Could you check a few things on this model? Use its own coordinates, in mm. A direction names the side the tool comes from. Give positions to 0.01 mm unless a question says otherwise; leave off trailing zeros. Loops run counter-clockwise (first coordinate to the right, second up) from the corner with the lowest first, then second, coordinate; pieces in that order, holes last. Notation, with made-up numbers: M 11,-9.5 L 70,-9.5 A8 cw 70,-2.5 Z; hole C 15.5,26.25 d2. An arc over 180 degrees is marked long. Answer in a Markdown table with one row per item. Add a question column.
```python
from build123d import *

# Parameters (mm, degrees)
BOSS_EXTRUDE5_DEPTH      = 6.35
FILLET1_R                = 25.4
CIRPATTERN7_COUNT        = 4
FILLET1_OF_CIRPATTERN7_R = 25.4
SKETCH13_R               = 15.556349186
BOSS_EXTRUDE8_DEPTH      = 6.35
SKETCH1_R                = 5.22699996
SKETCH1_R_2              = 1.686500056
CUT_EXTRUDE1_DEPTH       = 13.7


with BuildPart() as part:
    # Sketch4 → Boss-Extrude5 (new body)
    with BuildSketch(Plane(origin=(0, 0, 0), x_dir=(1, 0, 0), z_dir=(0, 1, 0))):
        Polygon((25.7955, 11), (25.7955, -11), (72.807954542, -58.012454542), (130.820409084, 0), (72.807954542, 58.012454542), align=None)
        Polygon((25.7955, 11), (14.7955, 0), (25.7955, -11), align=None)
        Polygon((25.7955, -11), (14.7955, 0), (25.7955, 11), (0, 11), (0, -11), align=None)
    boss_extrude5 = extrude(amount=BOSS_EXTRUDE5_DEPTH)

    # Fillet1
    fillet1_edges = [part.edges().sort_by_distance(p)[0] for p in [
        (130.820409084, 3.175, 0),
    ]]
    fillet(fillet1_edges, radius=FILLET1_R)

    # CirPattern7: Boss-Extrude5 ×4 about axis
    cirpattern7_axis = Axis((0, 0, 0), (0, 1, 0))
    for i in range(1, CIRPATTERN7_COUNT):
        add(boss_extrude5.rotate(cirpattern7_axis, i * 360 / CIRPATTERN7_COUNT))

    # Fillet1 of CirPattern7
    fillet1_of_cirpattern7_edges = [part.edges().sort_by_distance(p)[0] for p in [
        (0, 3.175, -130.820409084),
        (-130.820409084, 3.175, 0),
        (0, 3.175, 130.820409084),
    ]]
    fillet(fillet1_of_cirpattern7_edges, radius=FILLET1_OF_CIRPATTERN7_R)

    # Sketch13 → Boss-Extrude8 (add)
    with BuildSketch(Plane(origin=(0, 6.35, 0), x_dir=(1, 0, 0), z_dir=(0, 1, 0))):
        Circle(SKETCH13_R)
    extrude(amount=BOSS_EXTRUDE8_DEPTH)

    # Sketch1 → Cut-Extrude1 (cut, through all)
    with BuildSketch(Plane(origin=(0, 0, 0), x_dir=(1, 0, 0), z_dir=(0, 1, 0))):
        Circle(SKETCH1_R)
        with Locations((8.000000002, 0)):
            Circle(SKETCH1_R_2)
        with Locations((0, -8.000000002)):
            Circle(SKETCH1_R_2)
        with Locations((-8.000000002, 0)):
            Circle(SKETCH1_R_2)
        with Locations((0, 8.000000002)):
            Circle(SKETCH1_R_2)
    extrude(amount=CUT_EXTRUDE1_DEPTH, mode=Mode.SUBTRACT)


solid = part.part
```
Item 1: Suppose I cut it at D-D (x = 92.5). List the corners of the cut face in (y, z) for me, then the cut area to 3 significant figures.
Item 2: If we mould it in two halves opening along Z, with no side actions, what happens to faces 3 (the face through (38.27, 3.13, -92.55)), 4 (the face through (-11, 3, 18)), 5 (the face through (7, 12.7, 3))? For each: +Z half, -Z half, draft (parallel to the pull), parting line (faces both ways), or undercut.
Item 3: I need wall thicknesses on L1, parallel to Z at x = 0, y = 6.75; L2, parallel to X at y = 3.75, z = 0. Which ranges of each line are inside material? Lowest first, please.
Item 4: For P1, Ø3, axis at x = -19.5, y = 3.5, coming from the -Z side; P2, Ø5, axis at x = 18.5, y = 4, coming from the +Z side; P3, Ø1.9, axis at y = 3.5, z = 18.5, coming from the +X side; P4, Ø6, axis at x = -36, y = 10.5, coming from the -Z side, each with a flat end and sliding along its axis, tell me the tip position at first contact or that it passes through.
Item 5: Suppose I cut it at B-B (z = -52.5). List the corners of the cut face in (x, y) for me, then the cut area to 3 significant figures.
Item 6: Suppose I cut it at A-A (y = 3.5). Give the number of separate pieces and of enclosed holes in the cut face, then the cut area to 3 significant figures.
Item 7: Suppose I cut it at C-C (x = -44.5). List the corners of the cut face in (y, z) for me, then the cut area to 3 significant figures.
Item 8: For faces 1 (the face through (-0.279, 3.219, -120.298)), 2 (the face through (18, 3, 11)), which set-ups out of +Z, -Z, +X, -X, +Y, -Y let a thin tool reach every point of the face, with its end or its side?
Values found:
| question | item | result |
|---|---|---|
| 1 | outline | M 0,-38.32 L 6.35,-38.32 L 6.35,38.32 L 0,38.32 Z |
| 1 | area | 487 mm² |
| 2 | face 3 | -Z half |
| 2 | face 4 | undercut |
| 2 | face 5 | draft |
| 3 | L1 | -15.56 to -9.69, -6.31 to -5.23, 5.23 to 6.31, 9.69 to 15.56 |
| 3 | L2 | -120.3 to -9.69, -6.31 to -5.23, 5.23 to 6.31, 9.69 to 120.3 |
| 4 | P1 | z = -112.82 |
| 4 | P2 | z = 114.63 |
| 4 | P3 | x = 113.26 |
| 4 | P4 | through |
| 5 | outline | M -78.32,0 L -67.3,0 L -67.3,6.35 L -78.32,6.35 Z; M -37.7,0 L 37.7,0 L 37.7,6.35 L -37.7,6.35 Z; M 67.3,0 L 78.32,0 L 78.32,6.35 L 67.3,6.35 Z |
| 5 | area | 619 mm² |
| 6 | separate pieces | 1 |
| 6 | enclosed holes | 5 |
| 6 | area | 27,600 mm² |
| 7 | outline | M 0,-86.32 L 6.35,-86.32 L 6.35,-59.3 L 0,-59.3 Z; M 0,-29.7 L 6.35,-29.7 L 6.35,29.7 L 0,29.7 Z; M 0,59.3 L 6.35,59.3 L 6.35,86.32 L 0,86.32 Z |
| 7 | area | 720 mm² |
| 8 | face 1 | -Z, +Y, -Y |
| 8 | face 2 | +Y, -Y |
